Autodesk Inventor part; units mm, degrees
ref_plane "YZ Plane" through (0, 0, 0) normal (1, 0, 0) x (0, 1, 0)
ref_plane "XZ Plane" through (0, 0, 0) normal (0, 1, 0) x (-1, 0, 0)
ref_plane "XY Plane" through (0, 0, 0) normal (0, 0, 1) x (1, 0, 0)
sketch "Sketch1" plane through (0, 0, 0) normal (0, 0, 1) x (1, 0, 0)
  circle A0 centre (0, 0) radius 6.35
  circle A1 centre (0, 0) radius 3
  dimension "d0" = 12.7
  dimension "d1" = 6
extrude "Extrusion1" add sketch "Sketch1" along normal blind 434 contours A0 | A1
sketch "Sketch2" plane through (0, 0, 434) normal (0, 0, 1) x (1, 0, 0)
  circle A0 centre (0, 0) radius 3
  dimension "d4" = 6
sketch "Sketch3" plane through (0, 0, 0) normal (0, 0, -1) x (-1, 0, 0)
  circle A0 centre (0, 0) radius 3
  dimension "d7" = 6
hole "Agujero1" at (0, 0, 434) direction (0, 0, -1) diameter 6 depth 25 tip angle 120
hole "Agujero2" at (0, 0, 0) direction (0, 0, 1) diameter 6 depth 20 tip angle 118
thread "Rosca3"
thread "Rosca4"
sketch "Sketch4" plane through (0, 0, 434) normal (0, 0, 1) x (1, 0, 0)
  circle A0 centre (0, 0) radius 4
  circle A1 centre (0, 0) radius 6.5
  dimension "d32" = 8
  dimension "d38" = 13
extrude "Extrusion4" cut sketch "Sketch4" against normal blind 12
sketch "Sketch5" plane through (0, 0, 0) normal (0, 0, -1) x (-1, 0, 0)
  circle A0 centre (0, 0) radius 4
  circle A1 centre (0, 0) radius 6.5
  dimension "d35" = 8
  dimension "d39" = 13
extrude "Extrusion5" cut sketch "Sketch5" against normal blind 12
properties part number "Guías de Vínculo Cabezal" material "Steel, High Strength, Low Alloy"
The model under review builds one solid part; all positions refer to its coordinate system, in mm. A direction names the side the tool comes from. Round coordinates to 2 decimals unless told otherwise and drop trailing zeros. Order: outer loops, then holes, each group sorted by start corner. A loop starts at its lowest first (then second) coordinate and runs counter-clockwise, first axis right, second up. Notation, with made-up numbers: (29, 32.5) - (55, 32.5) arc R20 cw to (55, 45.5) - close; hole circle Ø1 at (28, 45). An arc over 180 degrees is marked (long way). Answer in a Markdown table with one row per item.
(1) For line 1 (Y direction, x = 0, z = 15.5); line 2 (Y direction, x = 0, z = 423.5); line 3 (Z direction, x = -5, y = 3.25), list the stretches that pass through material, from the lowest coordinate up. Write a range as from..to.
Result set:
| item | result |
|---|---|
| line 1 | y = -6.35..-3, 3..6.35 |
| line 2 | y = -4..-3, 3..4 |
| line 3 | z = 12..422 |
(2) Take a section at A-A on z = 229. Write out the cut boundary in (x, y).
Result set:
| item | result |
|---|---|
| outline | circle Ø12.7 at (0, 0) |
(3) Machinability: for faces 1 (the face through (1, 3, 0)), 2 (the face through (-1.3, -4.1, 12)), 3 (the face through (1.3, -4.1, 422)), which of the approach directions +Z, -Z, +X, -X, +Y, -Y give a long, thin tool a straight path to every point of the face, cutting with its end or side? Answer none if there is none.
Result set:
| item | result |
|---|---|
| face 1 | -Z, +X, -X, +Y, -Y |
| face 2 | -Z |
| face 3 | +Z |
(4) Clearance check with flat-ended pins moving along their axes: P1, Ø5, axis at y = 3.5, z = 76, coming from the -X side; P2, Ø7, axis at x = 0, y = 0, coming from the +Z side; P3, Ø1, axis at x = -2, y = 4.5, coming from the -Z side; P4, Ø1, axis at x = 1, z = 336.5, coming from the +Y side. State where each tip first meets the part, or that it passes through.
Result set:
| item | result |
|---|---|
| P1 | stops at x = -6.27 |
| P2 | stops at z = 434 |
| P3 | stops at z = 12 |
| P4 | stops at y = 6.33 |
